```python
from build123d import *

# Parameters (mm, degrees)
F0_R     = 1.984375
F1_DEPTH = 17.4625
F2_R     = 5.08


with BuildPart() as f1:
    # F0 (on Front) → F1 (new body)
    with BuildSketch(Plane.XZ):
        with BuildLine():
            Line((61.9125, 812.8), (25.4, 812.8))
            ThreePointArc((25.4, 812.8), (7.439488, 805.360512), (0, 787.4))
            Line((0, 787.4), (0, 762))
            Line((0, 762), (12.491861, 12.488363))
            ThreePointArc((12.491861, 12.488363), (16.28498, 3.645228), (25.190097, 0))
            Line((25.190097, 0), (62.122403, 0))
            ThreePointArc((62.122403, 0), (71.02752, 3.645228), (74.820639, 12.488363))
            Line((74.820639, 12.488363), (87.3125, 762))
            Line((87.3125, 762), (87.3125, 787.4))
            ThreePointArc((87.3125, 787.4), (79.873012, 805.360512), (61.9125, 812.8))
        make_face()
        with Locations((43.65625, 38.1)):
            Circle(F0_R, mode=Mode.SUBTRACT)
        with Locations((43.65625, 419.1)):
            Circle(F0_R, mode=Mode.SUBTRACT)
    extrude(amount=F1_DEPTH)

    # F2
    f2_edges = [f1.edges().sort_by_distance(p)[0] for p in [
        (6.24593, -17.4625, 387.244181),
        (7.439488, -17.4625, 805.360512),
    ]]
    fillet(f2_edges, radius=F2_R)


solid = f1.part
```
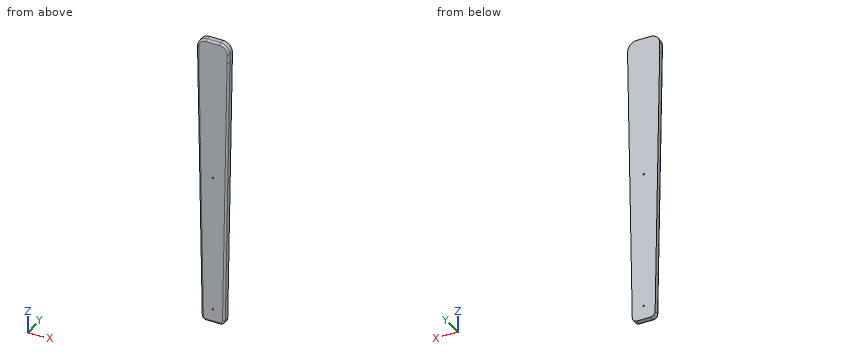
Verification items for the finished model (mm, model axes). Coordinates: 2 decimals unless noted, no trailing zeros. Order: outer loops, then holes, each group sorted by start corner. A loop starts at its lowest first (then second) coordinate and runs counter-clockwise, first axis right, second up. Notation, with made-up numbers: (79, 76.5) -> (130, 76.5) arc R33 ccw to (130, 107.5) -> close; hole circle Ø9 at (5.25, -38). An arc over 180 degrees is marked (long way). Answer as CSV lines item,"result". Start each with the question number.
1) Cross-section at A-A, the plane y = -4. Record the boundary of the cut face in (x, z), then the cut area to 3 significant figures.
2) Gauge pin test, flat ends, axial feed: pin 1 Ø5 at (x, z) = (43.66, 38.1) entering from -Y; pin 2 Ø1 at (y, z) = (-6.5, 135.5) entering from +X; pin 3 Ø6 at (y, z) = (-3.5, 693.5) entering from -X; pin 4 Ø1.5 at (x, y) = (66.5, -15.5) entering from -Z. Record the tip position at first contact, or that the pin passes through.
3) Material ranges on L1, parallel to Z at x = 43, y = -6; L2, parallel to Z at x = 45, y = -10.5; L3, parallel to Z at x = 64, y = -10.5, recorded low to high. Write a range as [from, to].
Conclusion:
1,outline,"(0, 762) -> (12.49, 12.49) arc R12.7 ccw to (25.19, 0) -> (62.12, 0) arc R12.7 ccw to (74.82, 12.49) -> (87.31, 762) -> (87.31, 787.4) arc R25.4 ccw to (61.91, 812.8) -> (25.4, 812.8) arc R25.4 ccw to (0, 787.4) -> close; hole circle Ø3.97 at (43.66, 38.1); hole circle Ø3.97 at (43.66, 419.1)"
1,area,"60,900 mm²"
2,pin 1,"stops at y = -17.46"
2,pin 2,"stops at x = 76.88"
2,pin 3,"stops at x = 1.09"
2,pin 4,"stops at z = 1.32"
3,L1,"z = [0, 36.23], [39.97, 417.23], [420.97, 812.8]"
3,L2,"z = [0, 36.64], [39.56, 417.64], [420.56, 812.8]"
3,L3,"z = [0.14, 812.71]"
